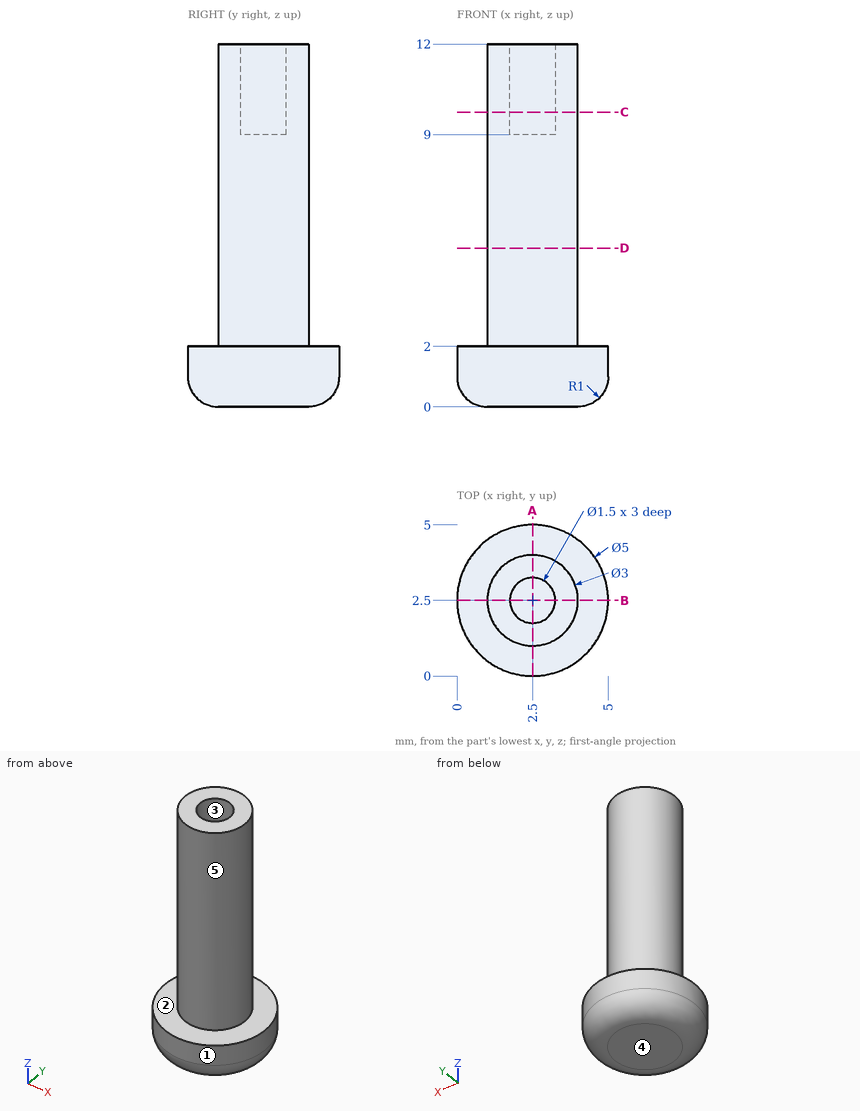
Could you check a few things on this drawing? It's one solid part, dimensions in mm from its lowest x, y, z. A direction names the side the tool comes from. Coordinates: 2 decimals unless noted, no trailing zeros. Write each loop counter-clockwise with the first axis right and the second up, starting at its lowest first coordinate (ties: lowest second). Pieces come first, ordered by that corner, then holes. Notation, with made-up numbers: (73, -37) - (120, -37) arc R32 ccw to (120, -4) - close; hole circle Ø11 at (80.5, 2). An arc over 180 degrees is marked (long way). Write item = value, one per line.
1) Suppose I cut it at A-A on x = 2.5. Please give me the cut outline in (y, z).
Result set:
outline = (0, 1) arc R1 ccw to (1, 0) - (4, 0) arc R1 ccw to (5, 1) - (5, 2) - (4, 2) - (4, 12) - (3.25, 12) - (3.25, 9) - (1.75, 9) - (1.75, 12) - (1, 12) - (1, 2) - (0, 2) - close
2) Please list where these lines run through material, in increasing order: line 1 (Y direction, x = 2.5, z = 10.35); line 2 (Y direction, x = 3.8, z = 2.25); line 3 (Y direction, x = 2.6, z = 5.75). Write a range as [from, to].
Result set:
line_1 = [1, 1.75], [3.25, 4]
line_2 = [1.75, 3.25]
line_3 = [1, 4]
3) We'd pull the mould along Y, two halves only. Please class the marked faces 1, 2 and 3: +Y half, -Y half, draft (parallel to the pull), parting line (faces both ways), or undercut.
Result set:
face_1 = parting line
face_2 = draft
face_3 = undercut
4) Suppose I cut it at D-D on z = 5.25. Please give me the cut outline in (x, y), plus the area to 3 significant figures.
Result set:
outline = circle Ø3 at (2.5, 2.5)
area = 7.07 mm2
5) Suppose I cut it at C-C on z = 9.75. Please give me the cut outline in (x, y), plus the area to 3 significant figures.
Result set:
outline = circle Ø3 at (2.5, 2.5); hole circle Ø1.5 at (2.5, 2.5)
area = 5.30 mm2
6) Will these pins go through, and if not, where does the flat tip stop? pin 1 Ø2 at (x, z) = (3.5, 6.5) entering from -Y; pin 2 Ø1.5 at (y, z) = (1.5, 7.5) entering from +X; pin 3 Ø1.2 at (x, y) = (2.5, 2.5) entering from +Z.
Result set:
pin_1 = 1
pin_2 = 3.98
pin_3 = 9
7) For the marked faces 4 and 5, which set-ups out of +Z, -Z, +X, -X, +Y, -Y let a thin tool reach every point of the face, with its end or its side?
Result set:
face_4 = -Z, +X, -X, +Y, -Y
face_5 = +Z
